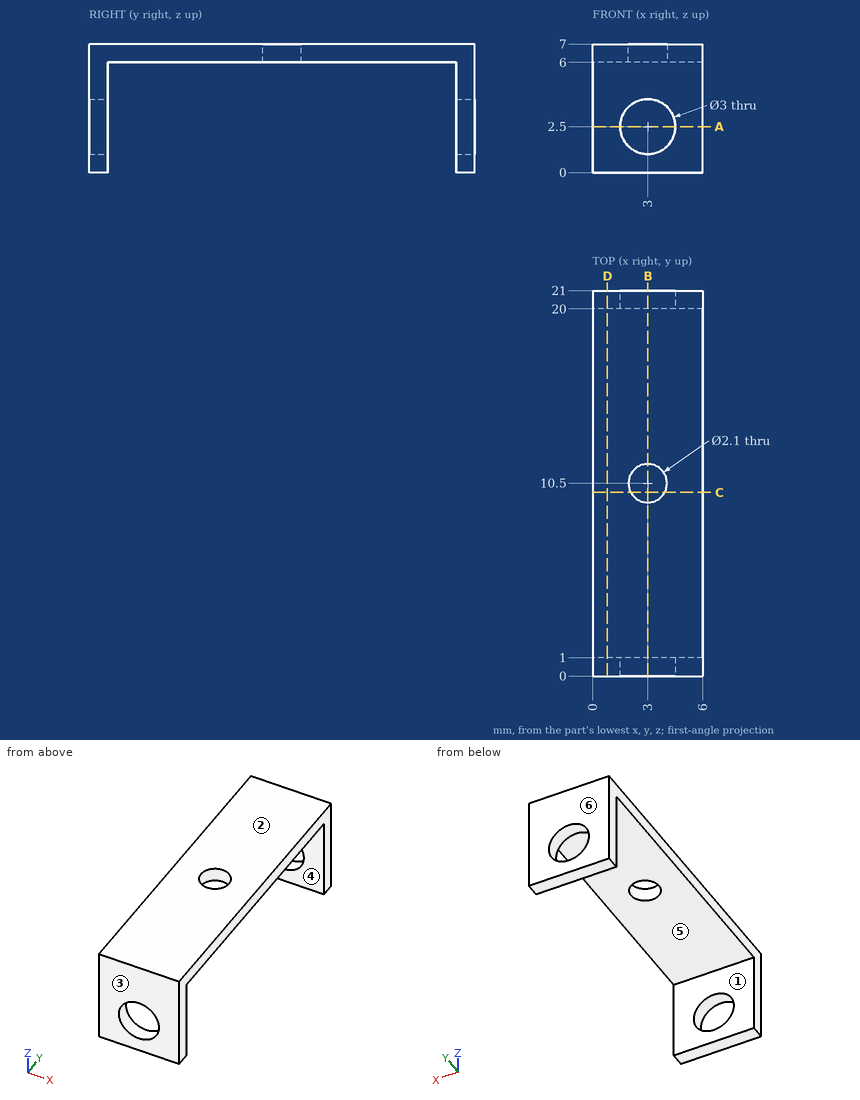
The figure shows three views and two pictorial views of one solid part (mm, origin at its lowest corner). Answer the questions. A direction names the side the tool comes from. Give positions to 0.01 mm unless a question says otherwise; leave off trailing zeros. Write each loop counter-clockwise with the first axis right and the second up, starting at its lowest first coordinate (ties: lowest second). Pieces come first, ordered by that corner, then holes. Notation, with made-up numbers: (-17, -14) - (40, -14) arc R18 ccw to (40, -9) - close; hole circle Ø1 at (32, 79). An arc over 180 degrees is marked (long way). Use one line per item in the form item = value.
1. For the marked faces 1 and 2, determine the directions among +Z, -Z, +X, -X, +Y, -Y from which every point of the face is accessible in a straight line to the end or side of a thin tool.
Filled in:
face_1 = -Z, +X, -X
face_2 = +Z, +X, -X, +Y, -Y
2. A cutting plane is placed at D-D (x = 0.8). Write down the section's boundary in (y, z), and give its area (3 significant figures).
Filled in:
outline = (0, 0) - (1, 0) - (1, 6) - (20, 6) - (20, 0) - (21, 0) - (21, 7) - (0, 7) - close
area = 33.0 mm^2
3. Consider L1, parallel to Y at x = 4.8, z = 5.5; L2, parallel to X at y = 20.55, z = 2.5; L3, parallel to Z at x = 3, y = 20.55. Determine where each line is inside the solid, lowest interval first.
Filled in:
L1 = 0 to 1, 20 to 21
L2 = 0 to 1.5, 4.5 to 6
L3 = 0 to 1, 4 to 7
4. A cutting plane is placed at C-C (y = 10). Write down the section's boundary in (x, z), and give its area (3 significant figures).
Filled in:
outline = (0, 6) - (2.08, 6) - (2.08, 7) - (0, 7) - close; (3.92, 6) - (6, 6) - (6, 7) - (3.92, 7) - close
area = 4.15 mm^2
5. Determine the mould class of the marked faces 3, 4, 5 and 6 for opening direction Y: released by +Y, released by -Y, zero draft, split by the parting line, or undercut.
Filled in:
face_3 = released by -Y
face_4 = undercut
face_5 = undercut
face_6 = released by +Y
6. Each of these flat-tipped pins is pushed along its axis until it touches: pin 1 Ø2 at (y, z) = (18.5, 6) entering from -X; pin 2 Ø1.8 at (x, y) = (2, 14.5) entering from -Z. Where does it stop, or does it pass through?
Filled in:
pin_1 = 0
pin_2 = 6
7. A cutting plane is placed at A-A (z = 2.5). Write down the section's boundary in (x, y).
Filled in:
outline = (0, 0) - (1.5, 0) - (1.5, 1) - (0, 1) - close; (0, 20) - (1.5, 20) - (1.5, 21) - (0, 21) - close; (4.5, 0) - (6, 0) - (6, 1) - (4.5, 1) - close; (4.5, 20) - (6, 20) - (6, 21) - (4.5, 21) - close
8. A cutting plane is placed at B-B (x = 3). Write down the section's boundary in (y, z), and give its area (3 significant figures).
Filled in:
outline = (0, 0) - (1, 0) - (1, 1) - (0, 1) - close; (0, 4) - (1, 4) - (1, 6) - (9.45, 6) - (9.45, 7) - (0, 7) - close; (11.55, 6) - (20, 6) - (20, 4) - (21, 4) - (21, 7) - (11.55, 7) - close; (20, 0) - (21, 0) - (21, 1) - (20, 1) - close
area = 24.9 mm^2
